Read the model definition and answer for the solid it produces. Units are mm, in the model's axes. Give positions to 0.01 mm unless a question says otherwise; leave off trailing zeros. Loops run counter-clockwise (first coordinate to the right, second up) from the corner with the lowest first, then second, coordinate; pieces in that order, holes last. Notation, with made-up numbers: (62.25, -31.5) - (114.25, -31.5) arc R12 cw to (114.25, -16.5) - close; hole circle Ø2 at (-37.5, 16). An arc over 180 degrees is marked (long way). Write each question's results on one line, items separated by ' | '. Start each with the question number.
Q1. The part is cut by section D-D, the plane x = 83. Write down the section's boundary in (y, z), plus the area to 3 significant figures.
Q2. The part is cut by section A-A, the plane y = 0. Write down the section's boundary in (x, z), plus the area to 3 significant figures.
Q3. Determine the mould class of faces 1 (the flat face through (-95, 0, 3)), 2 (the cylindrical face through (83.553, -4.214, 3.296)), 3 (the flat face through (95, 0, 3)), 4 (the flat face through (1, 20, 3)) for opening direction X: +X half, -X half, draft (parallel to the pull), parting line (faces both ways), or undercut.
Q4. Find the intervals of material crossed by line 1 (Y direction, x = 83, z = 3.75); line 2 (Y direction, x = -15, z = 6); line 3 (X direction, y = -3, z = 3.25), in increasing order. Write a range as from..to.
Q5. The part is cut by section C-C, the plane z = 3. Write down the section's boundary in (x, y), plus the area to 3 significant figures.
Q6. The part is cut by section B-B, the plane x = -15. Write down the section's boundary in (y, z).
Q7. Given pin 1 (1.5 mm diameter, centred on x = -37.5, y = -8.5, fed in from -Z), flat-ended and moving along its own axis, determine where the tip first touches the part or whether it passes through.
```python
from build123d import *

# Parameters (mm, degrees)
F1_DEPTH       = 6.5
F2_D           = 8.5
F3_D           = 8.5
F4_D           = 6.5
F4_CSINK_D     = 15
F4_CSINK_ANGLE = 82
F5_D           = 6.5
F5_CSINK_D     = 15
F5_CSINK_ANGLE = 82


with BuildPart() as f1:
    # F0 (on Top) → F1 (new body)
    with BuildSketch(Plane.XY):
        with BuildLine():
            Line((94, 20), (-94, 20))
            ThreePointArc((-94, 20), (-94.707107, 19.707107), (-95, 19))
            Line((-95, 19), (-95, -19))
            ThreePointArc((-95, -19), (-94.707107, -19.707107), (-94, -20))
            Line((-94, -20), (94, -20))
            ThreePointArc((94, -20), (94.707107, -19.707107), (95, -19))
            Line((95, -19), (95, 19))
            ThreePointArc((95, 19), (94.707107, 19.707107), (94, 20))
        make_face()
    extrude(amount=F1_DEPTH)

    # F2 (through all)
    with Locations(Plane(origin=(0, 0, 0), x_dir=(1, 0, 0), z_dir=(0, 0, -1))):
        with Locations((83, 0)):
            Hole(F2_D / 2)

    # F3 (through all)
    with Locations(Plane(origin=(0, 0, 0), x_dir=(1, 0, 0), z_dir=(0, 0, -1))):
        with Locations((-83, 0)):
            Hole(F3_D / 2)

    # F4 (through all)
    with Locations(Plane(origin=(0, 0, 0), x_dir=(1, 0, 0), z_dir=(0, 0, -1))):
        with Locations((15, 0)):
            CounterSinkHole(F4_D / 2, F4_CSINK_D / 2, counter_sink_angle=F4_CSINK_ANGLE)

    # F5 (through all)
    with Locations(Plane(origin=(0, 0, 0), x_dir=(1, 0, 0), z_dir=(0, 0, -1))):
        with Locations((-15, 0)):
            CounterSinkHole(F5_D / 2, F5_CSINK_D / 2, counter_sink_angle=F5_CSINK_ANGLE)


solid = f1.part
```
Check sheet entries:
1) outline: (-20, 0) - (-4.25, 0) - (-4.25, 6.5) - (-20, 6.5) - close; (4.25, 0) - (20, 0) - (20, 6.5) - (4.25, 6.5) - close | area: 205 mm^2
2) outline: (-95, 0) - (-87.25, 0) - (-87.25, 6.5) - (-95, 6.5) - close; (-78.75, 0) - (-22.5, 0) - (-18.25, 4.89) - (-18.25, 6.5) - (-78.75, 6.5) - close; (-11.75, 4.89) - (-7.5, 0) - (7.5, 0) - (11.75, 4.89) - (11.75, 6.5) - (-11.75, 6.5) - close; (18.25, 4.89) - (22.5, 0) - (78.75, 0) - (78.75, 6.5) - (18.25, 6.5) - close; (87.25, 0) - (95, 0) - (95, 6.5) - (87.25, 6.5) - close | area: 998 mm^2
3) face 1: -X half | face 2: undercut | face 3: +X half | face 4: draft
4) line 1: y = -20..-4.25, 4.25..20 | line 2: y = -20..-3.25, 3.25..20 | line 3: x = -95..-86.01, -79.99..-18.59, -11.41..11.41, 18.59..79.99, 86.01..95
5) outline: (-95, -19) arc R1 ccw to (-94, -20) - (94, -20) arc R1 ccw to (95, -19) - (95, 19) arc R1 ccw to (94, 20) - (-94, 20) arc R1 ccw to (-95, 19) - close; hole circle Ø8.5 at (-83, 0); hole circle Ø9.78 at (-15, 0); hole circle Ø9.78 at (15, 0); hole circle Ø8.5 at (83, 0) | area: 7,340 mm^2
6) outline: (-20, 0) - (-7.5, 0) - (-3.25, 4.89) - (-3.25, 6.5) - (-20, 6.5) - close; (3.25, 4.89) - (7.5, 0) - (20, 0) - (20, 6.5) - (3.25, 6.5) - close
7) pin 1: stops at z = 0
